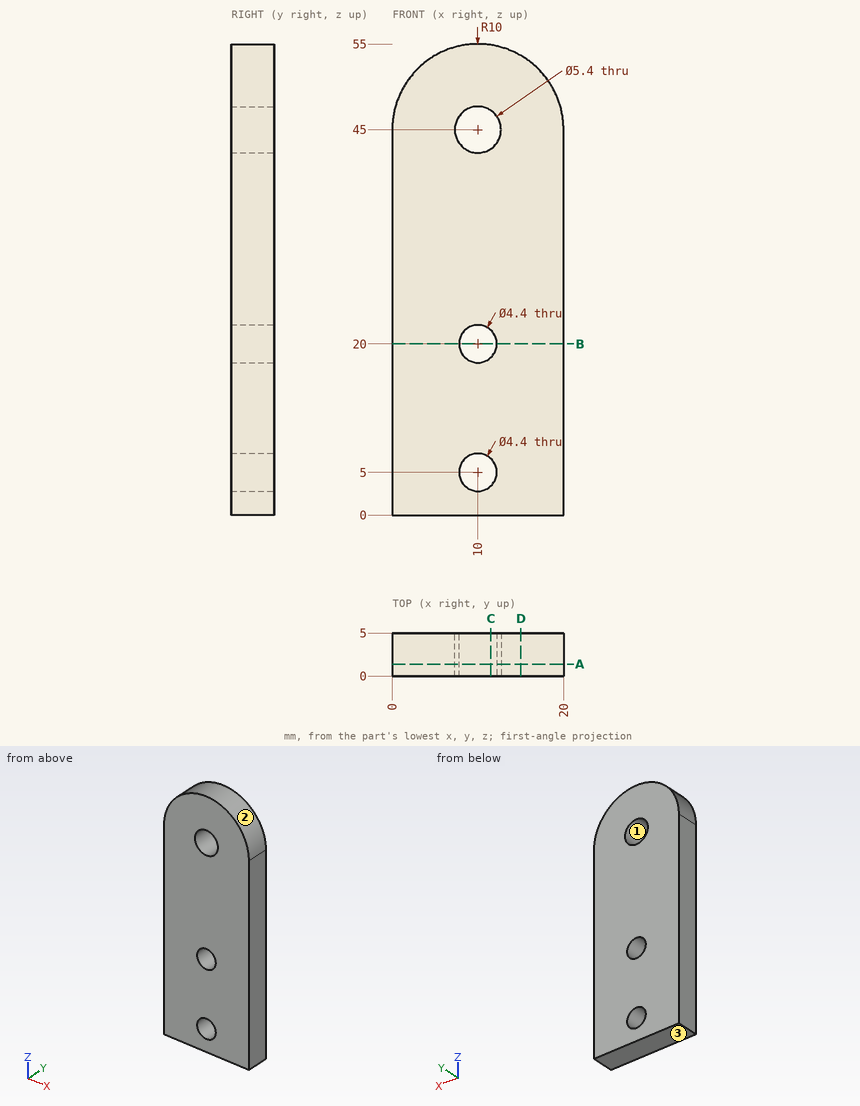
The drawing under review shows one solid part. Ordinate dimensions are in mm from its lowest x, y, z. Coordinates: 2 decimals unless noted, no trailing zeros. Order: outer loops, then holes, each group sorted by start corner. A loop starts at its lowest first (then second) coordinate and runs counter-clockwise, first axis right, second up. Notation, with made-up numbers: M -4,-6.75 L 45,-6.75 A11 cw 45,6.25 Z; hole C 23.25,9 d6. An arc over 180 degrees is marked long. Use a Markdown table: item, result.
(1) Add section C-C (x = 11.5). Give the boundary of the cut face in (y, z) (3 decimals), then the cut area to 3 significant figures.
Worked answers:
| item | result |
|---|---|
| outline | M 0,0 L 5,0 L 5,3.391 L 0,3.391 Z; M 0,6.609 L 5,6.609 L 5,18.391 L 0,18.391 Z; M 0,21.609 L 5,21.609 L 5,42.755 L 0,42.755 Z; M 0,47.245 L 5,47.245 L 5,54.887 L 0,54.887 Z |
| area | 220 mm2 |
(2) Wall thickness on probe 1 along Z at (x, y) = (10, 2.75); probe 2 along X at (y, z) = (4.8, 3.5); probe 3 along Z at (x, y) = (5, 1.6): over which ranges is each line inside the solid? List them lowest first.
Worked answers:
| item | result |
|---|---|
| probe 1 | z = 0 to 2.8, 7.2 to 17.8, 22.2 to 42.3, 47.7 to 55 |
| probe 2 | x = 0 to 8.39, 11.61 to 20 |
| probe 3 | z = 0 to 53.66 |
(3) Add section B-B (z = 20). Give the boundary of the cut face in (x, y).
Worked answers:
| item | result |
|---|---|
| outline | M 0,0 L 7.8,0 L 7.8,5 L 0,5 Z; M 12.2,0 L 20,0 L 20,5 L 12.2,5 Z |
(4) Add section D-D (x = 15). Give the boundary of the cut face in (y, z).
Worked answers:
| item | result |
|---|---|
| outline | M 0,0 L 5,0 L 5,53.66 L 0,53.66 Z |
(5) For P1, Ø4.5, axis at x = 10, z = 45, coming from the +Y side, flat-tipped, find the tip position at first contact; note if it passes through.
Worked answers:
| item | result |
|---|---|
| P1 | passes through |
(6) Draft analysis for pull direction Z (two halves, no side actions). For the marked faces 1, 2 and 3, state which applies: released by +Z, released by -Z, zero draft, split by the parting line, or undercut.
Worked answers:
| item | result |
|---|---|
| face 1 | undercut |
| face 2 | released by +Z |
| face 3 | released by -Z |
(7) Add section A-A (y = 1.4). Give the boundary of the cut face in (x, z), then the cut area to 3 significant figures.
Worked answers:
| item | result |
|---|---|
| outline | M 0,0 L 20,0 L 20,45 A10 ccw 0,45 Z; hole C 10,45 d5.4; hole C 10,5 d4.4; hole C 10,20 d4.4 |
| area | 1,000 mm2 |
